```python
from build123d import *

# Parameters (mm, degrees)
SKETCH1_W      = 41.91
SKETCH1_H      = 2.54
EXTRUDE1_DEPTH = 8.89
SKETCH2_R      = 0.254
EXTRUDE2_DEPTH = 1.27
SKETCH3_R      = 0.254
EXTRUDE3_DEPTH = 2.54


with BuildPart() as part:
    # Sketch1 → Extrude1 (new body)
    with BuildSketch(Plane(origin=(0, 0, 0), x_dir=(1, 0, 0), z_dir=(0, 1, 0))):
        Rectangle(SKETCH1_W, SKETCH1_H)
    extrude(amount=EXTRUDE1_DEPTH)

    # Sketch2 → Extrude2 (add)
    with BuildSketch(Plane(origin=(0, 0, 0), x_dir=(1, 0, 0), z_dir=(0, 1, 0))):
        with Locations(Location((19.05, 0, 0), (0, 0, 270))):
            Circle(SKETCH2_R)
        with Locations(Location((16.51, 0, 0), (0, 0, 270))):
            Circle(SKETCH2_R)
        with Locations(Location((13.97, 0, 0), (0, 0, 270))):
            Circle(SKETCH2_R)
        with Locations(Location((11.43, 0, 0), (0, 0, 270))):
            Circle(SKETCH2_R)
        with Locations(Location((8.89, 0, 0), (0, 0, 270))):
            Circle(SKETCH2_R)
        with Locations(Location((6.35, 0, 0), (0, 0, 270))):
            Circle(SKETCH2_R)
        with Locations(Location((3.81, 0, 0), (0, 0, 270))):
            Circle(SKETCH2_R)
        with Locations(Location((1.27, 0, 0), (0, 0, 270))):
            Circle(SKETCH2_R)
        with Locations(Location((-1.27, 0, 0), (0, 0, 270))):
            Circle(SKETCH2_R)
        with Locations(Location((-3.81, 0, 0), (0, 0, 270))):
            Circle(SKETCH2_R)
        with Locations(Location((-6.35, 0, 0), (0, 0, 270))):
            Circle(SKETCH2_R)
        with Locations(Location((-8.89, 0, 0), (0, 0, 270))):
            Circle(SKETCH2_R)
        with Locations(Location((-11.43, 0, 0), (0, 0, 270))):
            Circle(SKETCH2_R)
        with Locations(Location((-13.97, 0, 0), (0, 0, 270))):
            Circle(SKETCH2_R)
        with Locations(Location((-16.51, 0, 0), (0, 0, 270))):
            Circle(SKETCH2_R)
        with Locations(Location((-19.05, 0, 0), (0, 0, 270))):
            Circle(SKETCH2_R)
    extrude(amount=-EXTRUDE2_DEPTH)

    # Sketch3 → Extrude3 (cut)
    with BuildSketch(Plane(origin=(0, 8.89, 0), x_dir=(1, 0, 0), z_dir=(0, 1, 0))):
        with Locations(Location((6.35, 0, 0), (0, 0, 270))):
            Circle(SKETCH3_R)
        with Locations(Location((8.89, 0, 0), (0, 0, 270))):
            Circle(SKETCH3_R)
        with Locations(Location((11.43, 0, 0), (0, 0, 270))):
            Circle(SKETCH3_R)
        with Locations(Location((13.97, 0, 0), (0, 0, 270))):
            Circle(SKETCH3_R)
        with Locations(Location((16.51, 0, 0), (0, 0, 270))):
            Circle(SKETCH3_R)
        with Locations(Location((19.05, 0, 0), (0, 0, 270))):
            Circle(SKETCH3_R)
        with Locations(Location((-13.97, 0, 0), (0, 0, 270))):
            Circle(SKETCH3_R)
        with Locations(Location((-11.43, 0, 0), (0, 0, 270))):
            Circle(SKETCH3_R)
        with Locations(Location((-8.89, 0, 0), (0, 0, 270))):
            Circle(SKETCH3_R)
        with Locations(Location((-6.35, 0, 0), (0, 0, 270))):
            Circle(SKETCH3_R)
        with Locations(Location((-3.81, 0, 0), (0, 0, 270))):
            Circle(SKETCH3_R)
        with Locations(Location((-1.27, 0, 0), (0, 0, 270))):
            Circle(SKETCH3_R)
        with Locations(Location((1.27, 0, 0), (0, 0, 270))):
            Circle(SKETCH3_R)
        with Locations(Location((3.81, 0, 0), (0, 0, 270))):
            Circle(SKETCH3_R)
        with Locations(Location((-19.05, 0, 0), (0, 0, 270))):
            Circle(SKETCH3_R)
        with Locations(Location((-16.51, 0, 0), (0, 0, 270))):
            Circle(SKETCH3_R)
    extrude(amount=-EXTRUDE3_DEPTH, mode=Mode.SUBTRACT)


solid = part.part
```
Can you work these out from the model? Positions are in its coordinate system, mm. Round coordinates to 2 decimals unless told otherwise and drop trailing zeros. Loops run counter-clockwise (first coordinate to the right, second up) from the corner with the lowest first, then second, coordinate; pieces in that order, holes last.
Item 1: Suppose I cut it at B-B, the plane x = 2. Write out the boundary of the cut face in (y, z).
Item 2: Suppose I cut it at C-C, the plane z = 0.85. Write out the boundary of the cut face in (x, y) (3 decimals).
Item 3: Please list where these lines run through material, in increasing order: L1, parallel to Z at x = -19.05, y = 7.35; L2, parallel to Y at x = 16, z = 0.45.
Item 4: Will this pin go through, and if not, where does the flat tip stop? pin 1 Ø0.6 at (x, z) = (14, 0) entering from +Y.
Item 5: Suppose I cut it at A-A, the plane y = 8.25. State how many separate pieces and enclosed holes the cut face has, then the cut area to 3 significant figures.
Reported:
1. outline: (0, -1.27) - (8.89, -1.27) - (8.89, 1.27) - (0, 1.27) - close
2. outline: (-20.955, 0) - (20.955, 0) - (20.955, 8.89) - (-20.955, 8.89) - close
3. L1: z = -1.27 to -0.25, 0.25 to 1.27
3. L2: y = 0 to 8.89
4. pin 1: stops at y = 8.89
5. separate pieces: 1
5. enclosed holes: 16
5. area: 103 mm2
